Geometry: final body of the model. Coordinates: model frame, mm. Face numbers are marked on the shaded views. A direction names the side the tool comes from. Coordinates: 2 decimals unless noted, no trailing zeros. Order: outer loops, then holes, each group sorted by start corner. A loop starts at its lowest first (then second) coordinate and runs counter-clockwise, first axis right, second up. Notation, with made-up numbers: (-35.5, 44.5) -> (5.5, 44.5) arc R7 ccw to (5.5, 53.5) -> close; hole circle Ø7 at (-26, 8.25). An arc over 180 degrees is marked (long way). Use one line per item in the form item = value.
```python
from build123d import *

# Parameters (mm, degrees)
BOSS_EXTRUDE1_DEPTH = 25
CUT_EXTRUDE1_REACH  = 55.476
SKETCH2_R           = 3.25
SKETCH2_R_2         = 1.8
CUT_EXTRUDE2_REACH  = 60.206
SKETCH3_R           = 3


with BuildPart() as part:
    # Sketch1 → Boss-Extrude1 (new, symmetric)
    with BuildSketch(Plane(origin=(0, 0, 0), x_dir=(0, 0, -1), z_dir=(1, 0, 0))):
        with BuildLine():
            Line((0, 0), (0, 17))
            ThreePointArc((0, 17), (1.757359313, 21.242640687), (6, 23))
            Line((6, 23), (35.3, 23))
            ThreePointArc((35.3, 23), (37.421320344, 23.878679656), (38.3, 26))
            Line((38.3, 26), (38.3, 36))
            Line((38.3, 36), (41.3, 36))
            Line((41.3, 36), (41.3, 26))
            ThreePointArc((41.3, 26), (39.542640687, 21.757359313), (35.3, 20))
            Line((35.3, 20), (6, 20))
            ThreePointArc((6, 20), (3.878679656, 19.121320344), (3, 17))
            Line((3, 17), (3, 0))
            Line((3, 0), (0, 0))
        make_face()
    extrude(amount=BOSS_EXTRUDE1_DEPTH, both=True)

    # Sketch2 → Cut-Extrude1 (cut, up to next)
    with BuildSketch(Plane(origin=(0, 23, 0), x_dir=(1, 0, 0), z_dir=(0, 1, 0)), mode=Mode.PRIVATE) as cut_extrude1_sk1:
        with Locations(Location((0, 21.8, 0), (0, 0, 270))):
            Circle(SKETCH2_R)
    cut_extrude1_tool1 = extrude(cut_extrude1_sk1.sketch, amount=-CUT_EXTRUDE1_REACH, mode=Mode.PRIVATE) & part.part
    # Sketch2 → Cut-Extrude1 (cut, up to next)
    with BuildSketch(Plane(origin=(0, 23, 0), x_dir=(1, 0, 0), z_dir=(0, 1, 0)), mode=Mode.PRIVATE) as cut_extrude1_sk2:
        with Locations(Location((-18, 21.8, 0), (0, 0, 270))):
            Circle(SKETCH2_R_2)
    cut_extrude1_tool2 = extrude(cut_extrude1_sk2.sketch, amount=-CUT_EXTRUDE1_REACH, mode=Mode.PRIVATE) & part.part
    # Sketch2 → Cut-Extrude1 (cut, up to next)
    with BuildSketch(Plane(origin=(0, 23, 0), x_dir=(1, 0, 0), z_dir=(0, 1, 0)), mode=Mode.PRIVATE) as cut_extrude1_sk3:
        with Locations(Location((18, 21.8, 0), (0, 0, 270))):
            Circle(SKETCH2_R_2)
    cut_extrude1_tool3 = extrude(cut_extrude1_sk3.sketch, amount=-CUT_EXTRUDE1_REACH, mode=Mode.PRIVATE) & part.part
    add(cut_extrude1_tool1.solids().sort_by_distance((0, 23, -21.8))[0], mode=Mode.SUBTRACT)
    add(cut_extrude1_tool2.solids().sort_by_distance((-18, 23, -21.8))[0], mode=Mode.SUBTRACT)
    add(cut_extrude1_tool3.solids().sort_by_distance((18, 23, -21.8))[0], mode=Mode.SUBTRACT)

    # Sketch3 → Cut-Extrude2 (cut, up to next)
    with BuildSketch(Plane(origin=(0, 0, -3), x_dir=(-1, 0, 0), z_dir=(0, 0, -1)), mode=Mode.PRIVATE) as cut_extrude2_sk1:
        with Locations(Location((-17.5, 8, 0), (0, 0, 90))):
            Circle(SKETCH3_R)
    cut_extrude2_tool1 = extrude(cut_extrude2_sk1.sketch, amount=-CUT_EXTRUDE2_REACH, mode=Mode.PRIVATE) & part.part
    # Sketch3 → Cut-Extrude2 (cut, up to next)
    with BuildSketch(Plane(origin=(0, 0, -3), x_dir=(-1, 0, 0), z_dir=(0, 0, -1)), mode=Mode.PRIVATE) as cut_extrude2_sk2:
        with Locations(Location((17.5, 8, 0), (0, 0, 90))):
            Circle(SKETCH3_R)
    cut_extrude2_tool2 = extrude(cut_extrude2_sk2.sketch, amount=-CUT_EXTRUDE2_REACH, mode=Mode.PRIVATE) & part.part
    add(cut_extrude2_tool1.solids().sort_by_distance((17.5, 8, -3))[0], mode=Mode.SUBTRACT)
    add(cut_extrude2_tool2.solids().sort_by_distance((-17.5, 8, -3))[0], mode=Mode.SUBTRACT)


solid = part.part
```
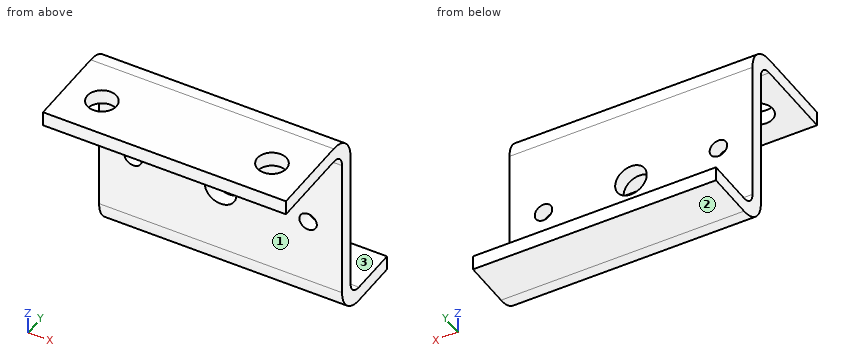
1) Contact query for flat-ended pins moving along their axis: P1, Ø3, axis at x = 18, z = -21.8, coming from the -Y side; P2, Ø7, axis at x = 17.5, y = 8, coming from the -Z side; P3, Ø7.5, axis at x = 0, z = -21.8, coming from the -Y side; P4, Ø23.5, axis at x = -2.5, z = -18.5, coming from the +Y side. Output: stop coordinate, or through.
Results found:
P1 = through
P2 = -3
P3 = 20
P4 = 23
2) Section B-B, the plane z = -21.8. Output: boundary loops of the cut face in (x, y), and give its area (3 significant figures).
Results found:
outline = (-25, 20) -> (-19.8, 20) -> (-19.8, 23) -> (-25, 23) -> close; (-16.2, 20) -> (-3.25, 20) -> (-3.25, 23) -> (-16.2, 23) -> close; (3.25, 20) -> (16.2, 20) -> (16.2, 23) -> (3.25, 23) -> close; (19.8, 20) -> (25, 20) -> (25, 23) -> (19.8, 23) -> close
area = 109 mm2
3) Section A-A, the plane x = 0. Output: boundary loops of the cut face in (y, z).
Results found:
outline = (0, -3) -> (17, -3) arc R3 cw to (20, -6) -> (20, -18.55) -> (23, -18.55) -> (23, -6) arc R6 ccw to (17, 0) -> (0, 0) -> close; (20, -35.3) arc R6 ccw to (26, -41.3) -> (36, -41.3) -> (36, -38.3) -> (26, -38.3) arc R3 cw to (23, -35.3) -> (23, -25.05) -> (20, -25.05) -> close
4) Access query for the marked faces 1, 2 and 3. Directions: +Z, -Z, +X, -X, +Y, -Y. A direction counts if a zero-diameter tool reaches every point of the face in a straight line with its end or side. Return the directions, or none.
Results found:
face_1 = -Z, +X, -X, -Y
face_2 = -Z, +X, -X, +Y, -Y
face_3 = +Z, +X, -X, +Y
5) Section D-D, the plane x = -5.5. Output: boundary loops of the cut face in (y, z).
Results found:
outline = (0, -3) -> (17, -3) arc R3 cw to (20, -6) -> (20, -35.3) arc R6 ccw to (26, -41.3) -> (36, -41.3) -> (36, -38.3) -> (26, -38.3) arc R3 cw to (23, -35.3) -> (23, -6) arc R6 ccw to (17, 0) -> (0, 0) -> close
6) Section C-C, the plane y = 8. Output: boundary loops of the cut face in (x, z), and give its area (3 significant figures).
Results found:
outline = (-25, -3) -> (-20.5, -3) -> (-20.5, 0) -> (-25, 0) -> close; (-14.5, -3) -> (14.5, -3) -> (14.5, 0) -> (-14.5, 0) -> close; (20.5, -3) -> (25, -3) -> (25, 0) -> (20.5, 0) -> close
area = 114 mm2
7) Material intervals for probe 1 along X at (y, z) = (22.25, -21.8); probe 2 along X at (y, z) = (8, -1.8); probe 3 along Y at (x, z) = (-6.5, -22.5), sorted ascending. Write a range as from..to.
Results found:
probe_1 = -25..-19.8, -16.2..-3.25, 3.25..16.2, 19.8..25
probe_2 = -25..-20.5, -14.5..14.5, 20.5..25
probe_3 = 20..23
